Autodesk Inventor part; units mm, degrees
ref_plane "YZ Plane" through (0, 0, 0) normal (1, 0, 0) x (0, 1, 0)
ref_plane "XZ Plane" through (0, 0, 0) normal (0, 1, 0) x (-1, 0, 0)
ref_plane "XY Plane" through (0, 0, 0) normal (0, 0, 1) x (1, 0, 0)
sketch "Boceto1" plane through (0, 0, 0) normal (0, 1, 0) x (-1, 0, 0)
  line L0 (19.05, -12.7) -> (-19.05, -12.7)
  line L1 (-19.05, -12.7) -> (-19.05, 12.7)
  line L2 (-19.05, 12.7) -> (19.05, 12.7)
  line L3 (19.05, 12.7) -> (19.05, -12.7)
  line L4 (19.05, -12.7) -> (-19.05, 12.7) construction
  line L5 (-19.05, -12.7) -> (19.05, 12.7) construction
  point P0 (0, 0)
  dimension "d0" = 38.1
  dimension "d1" = 25.4
extrude "Placa1" add sketch "Boceto1" along normal blind 0.45
sketch "Boceto2" plane through (-19.05, 0.45, 12.25) normal (0, 0, 1) x (1, 0, 0)
  line L0 (38.1, 0) -> (0, 0)
  line L1 (0, 0) -> (0, -9.525)
  line L2 (0, -9.525) -> (38.1, -9.525)
  line L3 (38.1, -9.525) -> (38.1, 0)
edge flange "Pestaña1" height 9.525 angle 90 thickness 0.45 bend radius 0.45 thickness toward (0, 0, 1) relief tear relief width 0.45 relief depth 0.225 corner gap 0.45 corner form 0 edges at (0, 0, 12.7) (0, 0, -12.7) wall of the first edge with corners at (19.05, 0.45, 12.25) (-19.05, 0.45, 12.25) (-19.05, -9.075, 12.25) (19.05, -9.075, 12.25)
bend "Doblez1"
corner "Esquina1"
fillet "Empalme1" radius 2 4 edges at (19.05, -9.075, 12.475) (19.05, -9.075, -12.475) (-19.05, -9.075, 12.475) (-19.05, -9.075, -12.475)
sketch "Boceto3" plane through (0, 0.45, 0) normal (0, 1, 0) x (1, 0, 0)
  circle A0 centre (0, 0) radius 3.175
  dimension "d14" = 6.35
extrude "Cortar1" cut sketch "Boceto3" against normal blind 0.45
equation "\"d15\" = Grosor"
equation "\"d2\" = Grosor"
equation "\"d3\" = Anchura_desahogo_plegado"
equation "\"d4\" = Profundidad_desahogo_plegado"
equation "\"d5\" = Remanente_mínimo"
equation "\"d6\" = Radiodetransición"
equation "\"d9\" = Radio_pliegue"
equation "\"d10\" = Tamaño_destalonado"
equation "\"d11\" = TamañoSeparación"
equation "\"d12\" = Tamaño_de_radio_de_Jacobi"
equation "\"Radio_pliegue\" = Grosor"
equation "\"Anchura_desahogo_plegado\" = Grosor"
equation "\"Profundidad_desahogo_plegado\" = 0.5 * Grosor"
equation "\"Tamaño_destalonado\" = 4 * Grosor"
equation "\"Remanente_mínimo\" = 2 * Grosor"
equation "\"Radiodetransición\" = Radio_pliegue"
equation "\"Tamaño_de_radio_de_Jacobi\" = Radio_pliegue"
equation "\"TamañoSeparación\" = Grosor"
properties part number "guarda_conector_ceramico" material "Acero AISI 1006 85 LC"
Can you work these out from the model? Positions are in its coordinate system, mm. A direction names the side the tool comes from. Coordinates: 2 decimals unless noted, no trailing zeros. Loops run counter-clockwise (first coordinate to the right, second up) from the corner with the lowest first, then second, coordinate; pieces in that order, holes last. Notation, with made-up numbers: M 81,29.25 L 126,29.25 A21 cw 126,57.25 Z; hole C 80,55.5 d6. An arc over 180 degrees is marked long. Put each result on its own line as item: value. Start each with the question number.
(1) Imagine slicing it at C-C on z = 0. List the corners of the cut face in (x, y) for me (3 decimals), and give its area (3 significant figures).
(2) I need wall thicknesses on probe 1 along X at (y, z) = (0.35, 0) (3 decimals); probe 2 along Z at (x, y) = (12.5, -7); probe 3 along Y at (x, z) = (-15.5, 10.25). Which ranges of each line are inside material? Lowest first, please.
(3) Will this pin go through, and if not, where does the flat tip stop? pin 1 Ø12 at (x, z) = (-3, -5) entering from -Y.
(4) Imagine slicing it at B-B on x = 0. List the corners of the cut face in (y, z) for me (3 decimals).
(5) Which directions (+Z, -Z, +X, -X, +Y, -Y) give clear straight access to the entire face, cutting with the end or side of a thin tool? Please do faces 1 (the face through (-18.449, -8.505, -12.478)), 2 (the face through (5, 0, 0)).
(6) Imagine slicing it at D-D on x = -11. List the corners of the cut face in (y, z) for me (3 decimals).
(7) We'd pull the mould along Z, two halves only. Please class faces 3 (the face through (0, -5, -12.25)), 4 (the face through (0, -5, -12.7)), 5 (the face through (-18.48, -8.474, 12.478)): +Z half, -Z half, draft (parallel to the pull), parting line (faces both ways), or undercut.
(8) Imagine slicing it at A-A on y = -2.5. List the corners of the cut face in (x, z) for me, and give its area (3 significant figures).
Worked answers:
1. outline: M -19.05,0 L -3.175,0 L -3.175,0.45 L -19.05,0.45 Z; M 3.175,0 L 19.05,0 L 19.05,0.45 L 3.175,0.45 Z
1. area: 14.3 mm2
2. probe 1: x = -19.05 to -3.175, 3.175 to 19.05
2. probe 2: z = -12.7 to -12.25, 12.25 to 12.7
2. probe 3: y = 0 to 0.45
3. pin 1: stops at y = 0
4. outline: M -9.075,-12.7 L -0.45,-12.7 A0.9 ccw 0.45,-11.8 L 0.45,-3.175 L 0,-3.175 L 0,-11.8 A0.45 cw -0.45,-12.25 L -9.075,-12.25 Z; M -9.075,12.25 L -0.45,12.25 A0.45 cw 0,11.8 L 0,3.175 L 0.45,3.175 L 0.45,11.8 A0.9 ccw -0.45,12.7 L -9.075,12.7 Z
5. face 1: +Z, -Z, -X, -Y
5. face 2: +X, -X, -Y
6. outline: M -9.075,-12.7 L -0.45,-12.7 A0.9 ccw 0.45,-11.8 L 0.45,11.8 A0.9 ccw -0.45,12.7 L -9.075,12.7 L -9.075,12.25 L -0.45,12.25 A0.45 cw 0,11.8 L 0,-11.8 A0.45 cw -0.45,-12.25 L -9.075,-12.25 Z
7. face 3: undercut
7. face 4: -Z half
7. face 5: draft
8. outline: M -19.05,-12.7 L 19.05,-12.7 L 19.05,-12.25 L -19.05,-12.25 Z; M -19.05,12.25 L 19.05,12.25 L 19.05,12.7 L -19.05,12.7 Z
8. area: 34.3 mm2
